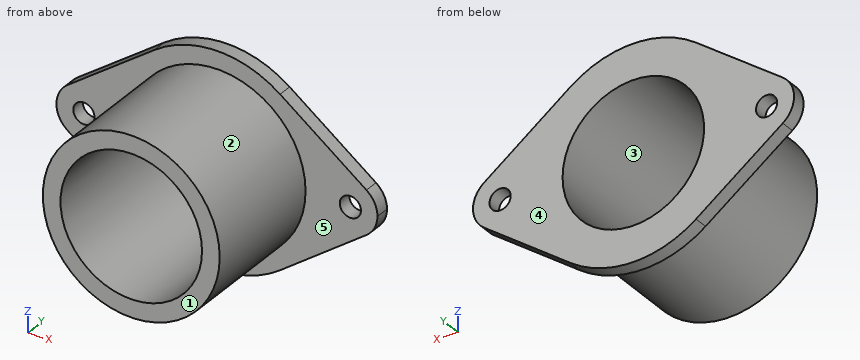
from build123d import *

# Parameters (mm, degrees)
F0_R     = 3.81
F0_R_2   = 31.75
F0_R_3   = 25.4
F1_DEPTH = 5.08
F2_R     = 31.75
F2_R_2   = 25.4
F3_DEPTH = 45.72


with BuildPart() as f1:
    # F0 (on Front) → F1 (new body)
    with BuildSketch(Plane.XZ):
        with BuildLine():
            Line((-22.499841, 30.746824), (-53.648159, 7.953178))
            ThreePointArc((-53.648159, 7.953178), (-57.6834, 0), (-53.648159, -7.953178))
            Line((-53.648159, -7.953178), (-22.499841, -30.746824))
            ThreePointArc((-22.499841, -30.746824), (0.062757, -38.099948), (22.601009, -30.672535))
            Line((22.601009, -30.672535), (53.598991, -7.831721))
            ThreePointArc((53.598991, -7.831721), (38.1, 0), (53.598991, 7.831721))
            Line((53.598991, 7.831721), (22.601009, 30.672535))
            ThreePointArc((22.601009, 30.672535), (0.062757, 38.099948), (-22.499841, 30.746824))
        make_face()
        with Locations((-47.8282, 0)):
            Circle(F0_R, mode=Mode.SUBTRACT)
        Circle(F0_R_2, mode=Mode.SUBTRACT)
        Circle(F0_R_2)
        Circle(F0_R_3, mode=Mode.SUBTRACT)
        with BuildLine():
            ThreePointArc((57.5564, 0), (56.510863, 4.387395), (53.598991, 7.831721))
            ThreePointArc((53.598991, 7.831721), (38.1, 0), (53.598991, -7.831721))
            ThreePointArc((53.598991, -7.831721), (56.510863, -4.387395), (57.5564, 0))
        make_face()
        with Locations((47.8282, 0)):
            Circle(F0_R, mode=Mode.SUBTRACT)
    extrude(amount=F1_DEPTH)

    # F2 (on face) → F3 (join)
    with BuildSketch(Plane.XZ.offset(5.08)):
        Circle(F2_R)
        Circle(F2_R_2, mode=Mode.SUBTRACT)
    extrude(amount=F3_DEPTH)


solid = f1.part
Build history of the part. All positions in model axes, mm. Face numbers are marked on the shaded views. A direction names the side the tool comes from. Coordinates: 2 decimals unless noted, no trailing zeros. Write each loop counter-clockwise with the first axis right and the second up, starting at its lowest first coordinate (ties: lowest second). Pieces come first, ordered by that corner, then holes. Notation, with made-up numbers: (-4, 85) -> (30, 85) arc R22 ccw to (30, 99) -> close; hole circle Ø11 at (3, -33). An arc over 180 degrees is marked (long way). Use CSV: the item, a comma, the result in double quotes. Start each with the question number.
Q1. Cut at D-D, the plane x = -35.5. List the corners of the cut face in (y, z), then the cut area to 3 significant figures.
Q2. Cut at C-C, the plane x = 24. List the corners of the cut face in (y, z).
Q3. Cut at A-A, the plane x = 0. List the corners of the cut face in (y, z).
Q4. Cut at B-B, the plane y = -20. List the corners of the cut face in (x, z).
Q5. 3-axis set-ups, long thin cutter, end or side, ignore diameter. For the marked faces 4 and 5: which of +Z, -Z, +X, -X, +Y, -Y reach the whole face in a straight line?
Q6. Drill centre lines: probe 1 along Y at (x, z) = (-32, -2); probe 2 along Z at (x, y) = (0, -31); probe 3 along X at (y, z) = (-4, 18). Where is each one in solid material? Low to high.
Q7. Pull direction Z, two halves, no side cores. Call the marked faces 1, 2 and 3: released by +Z, released by -Z, zero draft, split by the parting line, or undercut.
Q8. Flat gauge pins, fed straight in: pin 1 Ø4.5 at (x, z) = (-47.83, 0) entering from +Y; pin 2 Ø5 at (y, z) = (-15, 24) entering from -X; pin 3 Ø8 at (x, y) = (-10, -24.5) entering from +Z; pin 4 Ø8 at (y, z) = (-8, 10.5) entering from +X. Where does each tip first touch, or does it go through?
Checked values:
1,outline,"(-5.08, -21.23) -> (0, -21.23) -> (0, 21.23) -> (-5.08, 21.23) -> close"
1,area,"216 mm²"
2,outline,"(-50.8, -20.79) -> (-5.08, -20.79) -> (-5.08, -29.64) -> (0, -29.64) -> (0, -8.32) -> (-50.8, -8.32) -> close; (-50.8, 8.32) -> (0, 8.32) -> (0, 29.64) -> (-5.08, 29.64) -> (-5.08, 20.79) -> (-50.8, 20.79) -> close"
3,outline,"(-50.8, -31.75) -> (-5.08, -31.75) -> (-5.08, -38.1) -> (0, -38.1) -> (0, -25.4) -> (-50.8, -25.4) -> close; (-50.8, 25.4) -> (0, 25.4) -> (0, 38.1) -> (-5.08, 38.1) -> (-5.08, 31.75) -> (-50.8, 31.75) -> close"
4,outline,"circle Ø63.5 at (0, 0); hole circle Ø50.8 at (0, 0)"
5,face 4,"+Z, -Z, +X, -X, +Y"
5,face 5,"-Y"
6,probe 1,"y = -5.08 to 0"
6,probe 2,"z = -31.75 to -25.4, 25.4 to 31.75"
6,probe 3,"x = -39.92 to -17.92, 17.92 to 39.8"
7,face 1,"zero draft"
7,face 2,"split by the parting line"
7,face 3,"undercut"
8,pin 1,"passes through"
8,pin 2,"stops at x = -23.36"
8,pin 3,"stops at z = 31.18"
8,pin 4,"stops at x = 53.69"
